Answer from the drawing. Dimensions are ordinates in mm from the lowest x, y and z of the part. Round coordinates to 2 decimals unless told otherwise and drop trailing zeros. Loops run counter-clockwise (first coordinate to the right, second up) from the corner with the lowest first, then second, coordinate; pieces in that order, holes last. Notation, with made-up numbers: (14, 8.25) - (68, 8.25) arc R16 ccw to (68, 17.25) - close; hole circle Ø9 at (-26, -32). An arc over 180 degrees is marked (long way). Answer as CSV lines item,"result". Start each with the question number.
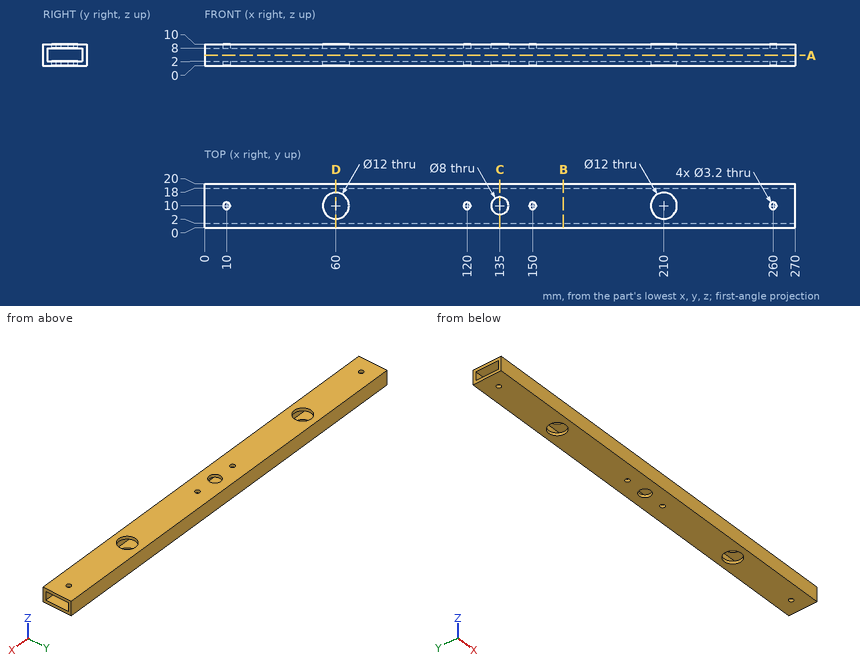
Item 1: Section A-A, the plane z = 4.75 is taken. Give the vertices of the cut face in (x, y).
Item 2: A flat-ended cylindrical pin translates along its axis: pin 1 Ø3 at (x, y) = (150, 10) entering from -Z. Find the tip coordinate at first contact, or state that the pin passes through.
Item 3: Section B-B, the plane x = 164 is taken. Give the vertices of the cut face in (y, z), and give its area (3 significant figures).
Item 4: Find the intervals of material crossed by L1, parallel to Z at x = 73.5, y = 13.5; L2, parallel to Y at x = 142.5, z = 5; L3, parallel to Y at x = 260, z = 8.7, in increasing order.
Item 5: Section D-D, the plane x = 60 is taken. Give the vertices of the cut face in (y, z).
Item 6: Section C-C, the plane x = 135 is taken. Give the vertices of the cut face in (y, z).
Answer:
1,outline,"(0, 0) - (270, 0) - (270, 2) - (0, 2) - close; (0, 18) - (270, 18) - (270, 20) - (0, 20) - close"
2,pin 1,"passes through"
3,outline,"(0, 0) - (20, 0) - (20, 10) - (0, 10) - close; hole (2, 2) - (18, 2) - (18, 8) - (2, 8) - close"
3,area,"104 mm²"
4,L1,"z = 0 to 2, 8 to 10"
4,L2,"y = 0 to 2, 18 to 20"
4,L3,"y = 0 to 8.4, 11.6 to 20"
5,outline,"(0, 0) - (4, 0) - (4, 2) - (2, 2) - (2, 8) - (4, 8) - (4, 10) - (0, 10) - close; (16, 0) - (20, 0) - (20, 10) - (16, 10) - (16, 8) - (18, 8) - (18, 2) - (16, 2) - close"
6,outline,"(0, 0) - (6, 0) - (6, 2) - (2, 2) - (2, 8) - (6, 8) - (6, 10) - (0, 10) - close; (14, 0) - (20, 0) - (20, 10) - (14, 10) - (14, 8) - (18, 8) - (18, 2) - (14, 2) - close"
